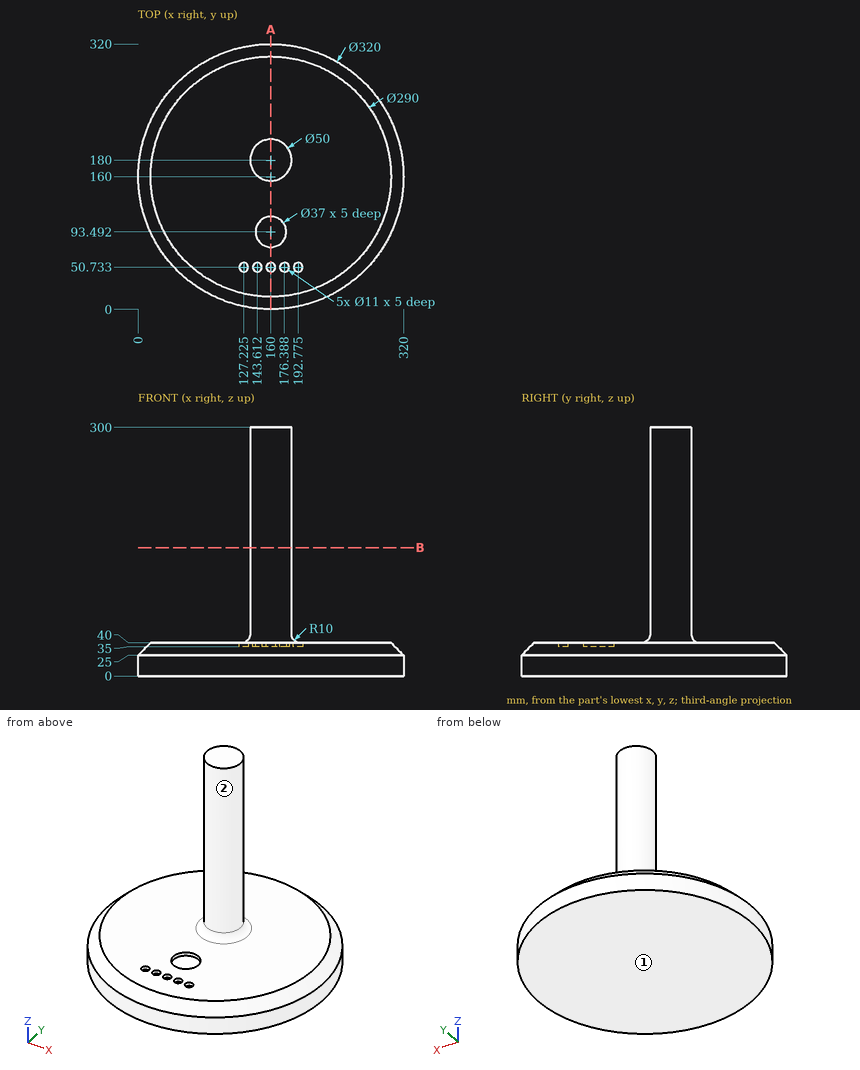
Geometry: see drawing. Coordinates: mm, zero at the bounding-box minimum. A direction names the side the tool comes from. Coordinates: 2 decimals unless noted, no trailing zeros. Write each loop counter-clockwise with the first axis right and the second up, starting at its lowest first coordinate (ties: lowest second). Pieces come first, ordered by that corner, then holes.
1) Section B-B on z = 155. Output: boundary loops of the cut face in (x, y), and give its area (3 significant figures).
2) Pin query (flat end, axial travel): pin 1 Ø11 at (x, y) = (153.5, 92.5) entering from +Z; pin 2 Ø1 at (y, z) = (228.5, 33) entering from -X (1 decimal); pin 3 Ø14.5 at (x, y) = (192.78, 50.73) entering from +Z. Return the tip coordinate at first contact, or that it passes through.
3) Material intervals for line 1 along X through (y, z) = (178, 180); line 2 along Z through (x, y) = (67, 254); line 3 along X through (y, z) = (169.5, 229.5), sorted ascending.
4) Section A-A on x = 160. Output: boundary loops of the cut face in (y, z), and give its area (3 significant figures).
5) Set-up query: the marked faces 1 and 2. Return all of +Z, -Z, +X, -X, +Y, -Y with unobstructed straight access to the full face (end or side cutting, diameter ignored); none if empty.
Check result:
1. outline: circle Ø50 at (160, 180)
1. area: 1,960 mm2
2. pin 1: stops at z = 35
2. pin 2: stops at x = 23.7
2. pin 3: stops at z = 40
3. line 1: x = 135.08 to 184.92
3. line 2: z = 0 to 40
3. line 3: x = 137.31 to 182.69
4. outline: (0, 0) - (320, 0) - (320, 25) - (305, 40) - (215, 40) arc R10 cw to (205, 50) - (205, 300) - (155, 300) - (155, 50) arc R10 cw to (145, 40) - (111.99, 40) - (111.99, 35) - (74.99, 35) - (74.99, 40) - (56.23, 40) - (56.23, 35) - (45.23, 35) - (45.23, 40) - (15, 40) - (0, 25) - close
4. area: 25,400 mm2
5. face 1: -Z, +X, -X, +Y, -Y
5. face 2: +Z
